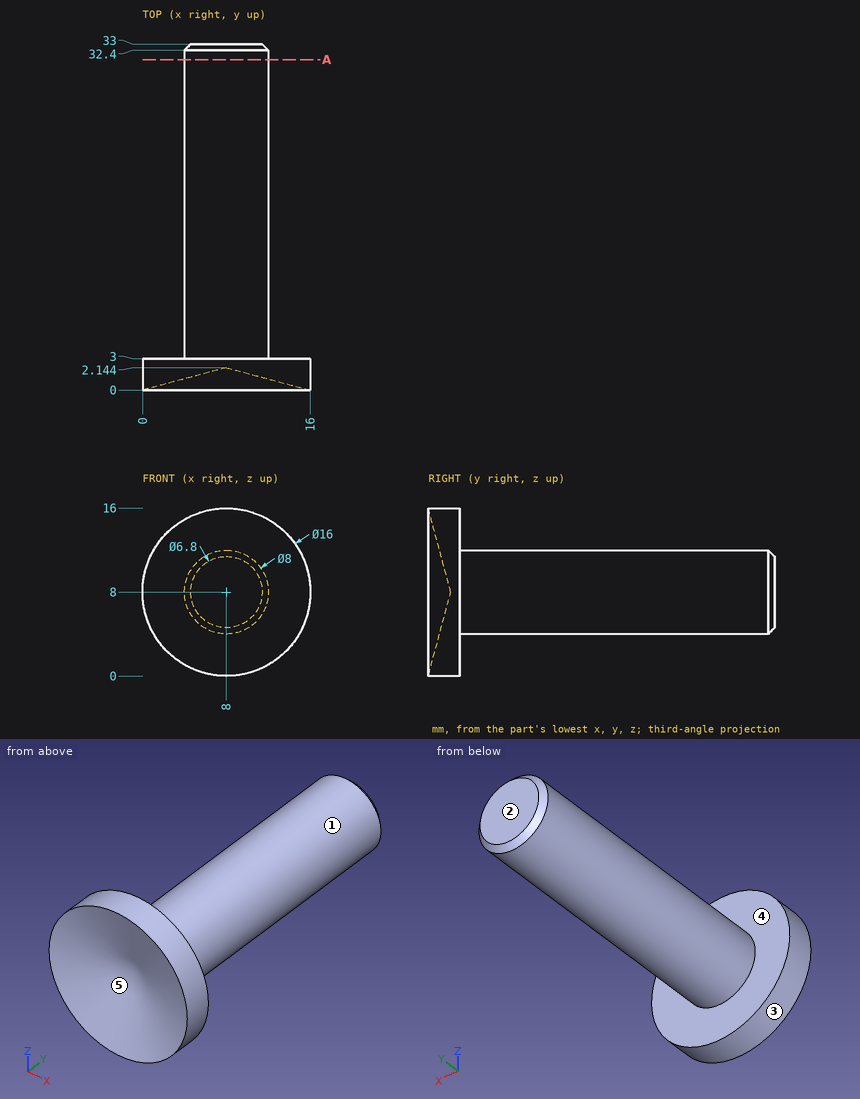
The figure shows three views and two pictorial views of one solid part (mm, origin at its lowest corner). Answer the questions. A direction names the side the tool comes from. Round coordinates to 2 decimals unless told otherwise and drop trailing zeros. Loops run counter-clockwise (first coordinate to the right, second up) from the corner with the lowest first, then second, coordinate; pieces in that order, holes last. Notation, with made-up numbers: M 53.5,-26.75 L 86.5,-26.75 A20 ccw 86.5,-4.75 Z; hole C -20.75,42 d2. An arc over 180 degrees is marked long. Return JSON: item names as keys, results as strings.
Q1. Find the intervals of material crossed by line 1 along Z through (x, y) = (7.75, 11); line 2 along Y through (x, z) = (9.25, 9.25); line 3 along Y through (x, z) = (4.25, 11), in increasing order. Write a range as from..to.
Results list:
{"line 1": "z = 4.01..11.99", "line 2": "y = 1.67..33", "line 3": "y = 0.86..3"}
Q2. Find section A-A, the plane y = 31.5. Determine the outline of the cut face in (x, z).
Results list:
{"outline": "C 8,8 d8"}
Q3. The mould has two halves that part along X. Classify the marked faces 3, 4 and 5: released by +X, released by -X, zero draft, split by the parting line, or undercut.
Results list:
{"face 3": "split by the parting line", "face 4": "zero draft", "face 5": "undercut"}
Q4. Which of the six approach directions +Z, -Z, +X, -X, +Y, -Y give full straight-line access (tool end or side, diameter ignored) to the marked faces 1 and 2?
Results list:
{"face 1": "+Y", "face 2": "+Z, -Z, +X, -X, +Y"}
Q5. Each of these flat-tipped pins is pushed along its axis until it touches: pin 1 Ø3 at (x, z) = (1.5, 14) entering from +Y; pin 2 Ø8 at (x, y) = (4.5, 21.5) entering from -Z; pin 3 Ø4 at (x, y) = (10.5, 6.5) entering from +Z; pin 4 Ø5 at (x, z) = (4.5, 10.5) entering from +Y. Where does it stop, or does it pass through?
Results list:
{"pin 1": "stops at y = 3", "pin 2": "stops at z = 4", "pin 3": "stops at z = 11.97", "pin 4": "stops at y = 33"}
